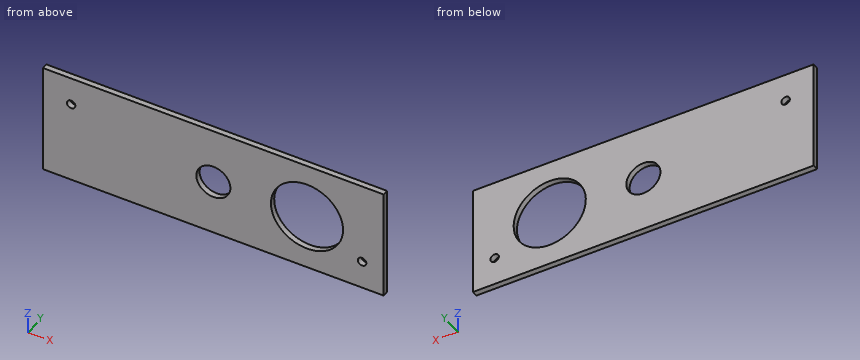
from build123d import *

# Parameters (mm, degrees)
SKETCH1_W           = 59.944
SKETCH1_H           = 20.066
SKETCH1_R           = 6.35
SKETCH1_R_2         = 0.75
SKETCH1_R_3         = 3
BOSS_EXTRUDE1_DEPTH = 1


with BuildPart() as part:
    # Sketch1 → Boss-Extrude1 (new body)
    with BuildSketch(Plane(origin=(0, 0, 0), x_dir=(1, 0, 0), z_dir=(0, 1, 0))):
        Rectangle(SKETCH1_W, SKETCH1_H)
        with Locations(Location((16.472, 0, 0), (0, 0, 270))):
            Circle(SKETCH1_R, mode=Mode.SUBTRACT)
        with Locations(Location((26.172, 4.9, 0), (0, 0, 270))):
            Circle(SKETCH1_R_2, mode=Mode.SUBTRACT)
        with Locations(Location((-25.028, -4.9, 0), (0, 0, 270))):
            Circle(SKETCH1_R_2, mode=Mode.SUBTRACT)
        with Locations(Location((0, 0, 0), (0, 0, 270))):
            Circle(SKETCH1_R_3, mode=Mode.SUBTRACT)
    extrude(amount=BOSS_EXTRUDE1_DEPTH)


solid = part.part
The listing builds one solid part. Answer for the finished solid, in the listing's coordinates (mm). Round coordinates to 2 decimals unless told otherwise and drop trailing zeros. Write each loop counter-clockwise with the first axis right and the second up, starting at its lowest first coordinate (ties: lowest second). Pieces come first, ordered by that corner, then holes. Notation, with made-up numbers: M 18.5,76 L 40.5,76 A29 cw 40.5,110 Z; hole C 29.5,-21.75 d2. An arc over 180 degrees is marked long. Write each question's results on one line, items separated by ' | '. Start each with the question number.
(1) The part is cut by section D-D, the plane x = 21. Write down the section's boundary in (y, z).
(2) The part is cut by section C-C, the plane y = 0.25. Write down the section's boundary in (x, z), and give its area (3 significant figures).
(3) Find the intervals of material crossed by line 1 (X direction, y = 0.35, z = 0); line 2 (X direction, y = 0.4, z = 4.9); line 3 (Z direction, x = 16.5, y = 0.25), in increasing order.
(4) The part is cut by section A-A, the plane x = 0. Write down the section's boundary in (y, z).
(5) This flat-tipped pin is pushed along its axis until it touches: P1, Ø1.4, axis at x = -25.028, z = 4.9, coming from the -Y side. Where does it stop, or does it pass through?
(6) The part is cut by section B-B, the plane z = 0. Write down the section's boundary in (x, y).
Worked answers:
1) outline: M 0,-10.03 L 1,-10.03 L 1,-4.45 L 0,-4.45 Z; M 0,4.45 L 1,4.45 L 1,10.03 L 0,10.03 Z
2) outline: M -29.97,-10.03 L 29.97,-10.03 L 29.97,10.03 L -29.97,10.03 Z; hole C -25.03,4.9 d1.5; hole C 0,0 d6; hole C 16.47,0 d12.7; hole C 26.17,-4.9 d1.5 | area: 1,040 mm²
3) line 1: x = -29.97 to -3, 3 to 10.12, 22.82 to 29.97 | line 2: x = -29.97 to -25.78, -24.28 to 12.43, 20.51 to 29.97 | line 3: z = -10.03 to -6.35, 6.35 to 10.03
4) outline: M 0,-10.03 L 1,-10.03 L 1,-3 L 0,-3 Z; M 0,3 L 1,3 L 1,10.03 L 0,10.03 Z
5) P1: passes through
6) outline: M -29.97,0 L -3,0 L -3,1 L -29.97,1 Z; M 3,0 L 10.12,0 L 10.12,1 L 3,1 Z; M 22.82,0 L 29.97,0 L 29.97,1 L 22.82,1 Z
